Could you check a few things on this model? Use its own coordinates, in mm. A direction names the side the tool comes from. Give positions to 0.01 mm unless a question says otherwise; leave off trailing zeros. Order: outer loops, then holes, each group sorted by start corner. A loop starts at its lowest first (then second) coordinate and runs counter-clockwise, first axis right, second up. Notation, with made-up numbers: (78, 26) - (89, 26) arc R29 cw to (89, 59) - close; hole circle Ø3 at (30.5, 55). An arc over 180 degrees is marked (long way). One line per question, with ' | ' between items. Start each with the question number.
1. Imagine slicing it at B-B (x = 168.5). Please give me the cut outline in (y, z), and give its area (3 significant figures).
2. Which directions (+Z, -Z, +X, -X, +Y, -Y) give clear straight access to the entire face, cutting with the end or side of a thin tool? Please do faces 1 (the flat face through (6.35, 61, -601)), 2 (the flat face through (474, 2, -1219.2)).
3. I need wall thicknesses on probe 1 along Z at (x, y) = (38, 2); probe 2 along Z at (x, y) = (25, 2); probe 3 along Z at (x, y) = (139, 4). Which ranges of each line are inside material? Lowest first, please. Write a range as from..to.
4. For P1, Ø8, axis at x = 526, z = -526, coming from the -Y side; P2, Ø10, axis at x = 637.5, z = -363, coming from the +Y side; P3, Ø8, axis at y = 43, z = -750.5, coming from the +X side, each with a flat end and sliding along its axis, tell me the tip position at first contact or that it passes through.
Autodesk Inventor part; units mm, degrees
ref_plane "YZ Plane" through (0, 0, 0) normal (1, 0, 0) x (0, 1, 0)
ref_plane "XZ Plane" through (0, 0, 0) normal (0, 1, 0) x (-1, 0, 0)
ref_plane "XY Plane" through (0, 0, 0) normal (0, 0, 1) x (1, 0, 0)
sketch "Sketch1" plane through (0, 0, 0) normal (0, 0, 1) x (1, 0, 0)
  line L0 (0, 114.3) -> (0, 4.7625)
  line L1 (4.7625, 0) -> (952.5, 0)
  line L2 (952.5, 0) -> (952.5, 6.35)
  line L3 (952.5, 6.35) -> (9.525, 6.35)
  line L4 (6.35, 9.525) -> (6.35, 114.3)
  line L5 (6.35, 114.3) -> (0, 114.3)
  arc A0 (6.35, 9.525) -> (9.525, 6.35) centre (9.525, 9.525) ccw
  arc A1 (0, 4.7625) -> (4.7625, 0) centre (4.7625, 4.7625) ccw
  point P0 (0, 0)
  dimension "d0" = 114.3
  dimension "d1" = 6.35
  dimension "d2" = 6.35
  dimension "d3" = 952.5
  dimension "d4" = 3.175
  dimension "d5" = 4.7625
extrude "Extrusion1" add sketch "Sketch1" against normal blind 1219.2
hole "Hole1" at (25.4, 6.35, -76.2) direction (0, -1, 0) diameter 6.731 end through all
pattern_linear "Rectangular Pattern1" count 4 spacing 355.6 along (0, 0, -1) of "Hole1"
hole "Hole2" at (38.1, 6.35, -25.4) direction (0, -1, 0) diameter 12.7 depth 25.4 tip angle 118
pattern_linear "Rectangular Pattern2" count 2 spacing 1168.4 along (0, 0, -1) of "Hole2"
hole "Hole3" at (139.7, 6.35, -25.4) direction (0, -1, 0) diameter 4.7625 depth 25.4 tip angle 118
pattern_linear "Rectangular Pattern3" count 2 spacing 1168.4 along (0, 0, -1) of "Hole3"
properties part number "GE-12062"
Results found:
1) outline: (0, -1219.2) - (6.35, -1219.2) - (6.35, 0) - (0, 0) - close | area: 7,740 mm2
2) face 1: +Z, -Z, +X, +Y | face 2: -Z, +X, -X, +Y, -Y
3) probe 1: z = -1219.2..-1200.15, -1187.45..-31.75, -19.05..0 | probe 2: z = -1219.2..-1146.34, -1139.66..-790.74, -784.06..-435.14, -428.46..-79.54, -72.86..0 | probe 3: z = -1219.2..-1196.08, -1191.52..-27.68, -23.12..0
4) P1: stops at y = 0 | P2: stops at y = 6.35 | P3: stops at x = 6.35
